Read the model definition and answer for the solid it produces. Units are mm, in the model's axes. A direction names the side the tool comes from. Give positions to 0.01 mm unless a question says otherwise; leave off trailing zeros. Write each loop counter-clockwise with the first axis right and the second up, starting at its lowest first coordinate (ties: lowest second). Pieces come first, ordered by that corner, then holes. Notation, with made-up numbers: (-28, 38.5) - (9, 38.5) arc R7 ccw to (9, 43.5) - close; hole circle Ø9 at (74.5, 78). An arc over 180 degrees is marked (long way). Answer as CSV lines item,"result".
Autodesk Inventor part; units mm, degrees
ref_plane "YZ Plane" through (0, 0, 0) normal (1, 0, 0) x (0, 1, 0)
ref_plane "XZ Plane" through (0, 0, 0) normal (0, 1, 0) x (-1, 0, 0)
ref_plane "XY Plane" through (0, 0, 0) normal (0, 0, 1) x (1, 0, 0)
sketch "Sketch1" plane through (0, 0, 0) normal (0, 0, 1) x (1, 0, 0)
  line L0 (-12.7529, 51.3281) -> (87.2471, 51.3281)
  line L1 (87.2471, 51.3281) -> (87.2471, -8.6719)
  line L2 (87.2471, -8.6719) -> (-12.7529, -8.6719)
  line L3 (-12.7529, -8.6719) -> (-12.7529, 51.3281)
  point P0 (0, 0)
  dimension "d0" = 100
  dimension "d1" = 60
extrude "Extrusion1" add sketch "Sketch1" along normal blind 40
shell "Shell1" thickness 2 removed faces 1 at (20.5805, 31.3281, 0)
sketch "Sketch2" plane through (85.2471, -6.6719, 38) normal (0, 0, -1) x (-1, 0, 0)
  line L0 (0, 0) -> (0, 56)
  line L1 (43.2, 19) -> (43.2, 37)
  line L2 (0, 37) -> (0, 19)
  line L3 (43.2, 19) -> (40.7, 19)
  line L4 (40.7, 19) -> (40.7, 22.5)
  line L5 (0, 16.6053) -> (0, 19)
  line L6 (0, 19) -> (2.5, 19)
  line L7 (2.5, 19) -> (2.5, 22.5)
  line L8 (2.5, 22.5) -> (40.7, 22.5)
  line L9 (0, 19) -> (2.5, 19)
  line L10 (40.7, 19) -> (43.2, 19)
  line L11 (43.2, 37) -> (40.7, 37)
  line L12 (40.7, 37) -> (40.7, 33.5)
  line L13 (40.7, 33.5) -> (2.5, 33.5)
  line L14 (2.5, 33.5) -> (2.5, 37)
  line L15 (43.2, 37) -> (40.7, 37)
  line L16 (2.5, 37) -> (0, 37)
  line L17 (96, 0) -> (0, 0)
  circle A0 centre (41.92, 20.3797) radius 0.9
  circle A1 centre (41.95, 35.62) radius 0.9
  circle A2 centre (1.28, 20.38) radius 0.9
  circle A3 centre (1.25, 35.62) radius 0.9
  line L18 (0, 56) -> (96, 56)
  point P0 (85.2471, 6.6719)
  point P1 (1.25, 19)
  point P2 (41.95, 19)
  point P3 (0, 37)
  point P4 (1.25, 37)
  point P5 (1.25, 19)
  dimension "d5" = 43.2
  dimension "d6" = 18
  dimension "d7" = 2.5
  dimension "d8" = 3.5
  dimension "d9" = 2.5
  dimension "d10" = 3.5
  dimension "d12" = 3.5
  dimension "d13" = 1.8
  dimension "d14" = 1.38
  dimension "d15" = 1.28
  dimension "d16" = 1.8
  dimension "d17" = 1.8
  dimension "d18" = 1.8
  dimension "d19" = 1.38
  dimension "d20" = 1.28
  dimension "d29" = 1.38
  dimension "d30" = 1.25
  dimension "d31" = 3.5
  dimension "d32" = 19
  dimension "d33" = 1.38
extrude "Extrusion2" add sketch "Sketch2" along normal blind 25
sketch "Sketch5" plane through (85.2471, -6.6719, 38) normal (0, 0, -1) x (-1, 0, 0)
  line L0 (0, 56) -> (96, 56)
  line L1 (77.9752, 56) -> (75.9752, 56)
  line L2 (75.9752, 56) -> (75.9752, 36)
  line L3 (75.9752, 36) -> (77.9752, 36)
  line L4 (77.9752, 36) -> (77.9752, 56)
  point P0 (85.2471, 6.6719)
  point P1 (75.9752, 56)
  dimension "d40" = 20
  dimension "d41" = 2
extrude "Extrusion5" add sketch "Sketch5" along normal blind 20
sketch "Sketch6" plane through (-12.7529, -8.6719, 0) normal (-1, 0, 0) x (0, 0, 1)
  circle A0 centre (27, 48) radius 3.5
  line L0 (18, 58) -> (18, 31.1645)
  line L1 (13, 23.2797) -> (38, 23.2797)
  line L2 (0, 58) -> (38, 58)
  point P0 (0, 8.6719)
  point P1 (18, 44.5822)
  dimension "d44" = 7
  dimension "d45" = 9
  dimension "d46" = 10
extrude "Extrusion6" cut sketch "Sketch6" against normal blind 4
sketch "Sketch7" plane through (-10.7529, -6.6719, 0) normal (1, 0, 0) x (0, 0, -1)
  circle A0 centre (-27, 46) radius 4.5
  line L0 (-40, -2) -> (-40, 58)
  circle A1 centre (-27, 46) radius 3.5
  line L1 (0, 56) -> (-38, 56)
  point P0 (0, 6.6719)
  dimension "d49" = 9
  dimension "d50" = 13
  dimension "d51" = 7
  dimension "d52" = 10
extrude "Extrusion7" add sketch "Sketch7" along normal blind 14
sketch "Sketch8" plane through (85.2471, -6.6719, 38) normal (0, 0, -1) x (-1, 0, 0)
  line L0 (96, 56) -> (96, 0)
  line L1 (96, 20.025) -> (76, 20.025)
  line L2 (76, 20.025) -> (76, 18.025)
  line L3 (76, 18.025) -> (96, 18.025)
  line L4 (96, 18.025) -> (96, 20.025)
  line L5 (96, 0) -> (0, 0)
  point P0 (85.2471, 6.6719)
  dimension "d55" = 20
  dimension "d56" = 2
  dimension "d57" = 18.025
extrude "Extrusion8" add sketch "Sketch8" along normal blind 20
sketch "Sketch9" plane through (-12.7529, -8.6719, 0) normal (0, -1, 0) x (1, 0, 0)
  circle A0 centre (12, 27) radius 3.5
  line L0 (0, 40) -> (100, 40)
  line L1 (2, 0) -> (2, 38)
  point P0 (12.7529, 0)
  dimension "d60" = 7
  dimension "d61" = 13
  dimension "d62" = 10
extrude "Extrusion9" cut sketch "Sketch9" against normal blind 4
sketch "Sketch10" plane through (-10.7529, -6.6719, 0) normal (0, 1, 0) x (1, 0, 0)
  circle A0 centre (10, -27) radius 3.5
  line L0 (98, -40) -> (-2, -40)
  line L1 (-2, 0) -> (-2, -40)
  circle A1 centre (10, -27) radius 4.5
  point P0 (10.7529, 0)
  dimension "d65" = 7
  dimension "d66" = 13
  dimension "d67" = 12
  dimension "d68" = 9
extrude "Extrusion10" add sketch "Sketch10" along normal blind 14
sketch "Sketch11" plane through (87.2471, -8.6719, 0) normal (1, 0, 0) x (0, 0, -1)
  line L0 (-5, 25.8) -> (-10, 25.8)
  line L1 (-10, 25.8) -> (-10, 34.2)
  line L2 (-10, 34.2) -> (-5, 34.2)
  line L3 (-5, 34.2) -> (-5, 25.8)
  line L4 (-40, 0) -> (-40, 60)
  line L5 (0, 0) -> (-40, 0)
  point P0 (0, 8.6719)
  dimension "d71" = 5
  dimension "d72" = 8.4
  dimension "d73" = 30
  dimension "d74" = 25.8
extrude "Extrusion11" cut sketch "Sketch11" against normal blind 2
sketch "Sketch12" plane through (85.2471, -6.6719, 38) normal (0, 0, -1) x (-1, 0, 0)
  line L0 (96, 0) -> (0, 0)
  line L1 (96, 0) -> (93, 0)
  line L2 (93, 0) -> (93, 1)
  line L3 (95, 3) -> (96, 3)
  line L4 (96, 3) -> (96, 0)
  line L5 (96, 56.0056) -> (93, 56.0056)
  line L6 (93, 56.0056) -> (93, 55.0056)
  line L7 (95, 53.0056) -> (96, 53.0056)
  line L8 (96, 53.0056) -> (96, 56.0056)
  line L9 (0, 56.0056) -> (3, 56.0056)
  line L10 (3, 56.0056) -> (3, 55.0056)
  line L11 (1, 53.0056) -> (0, 53.0056)
  line L12 (0, 53.0056) -> (0, 56.0056)
  line L13 (0, 0) -> (3, 0)
  line L14 (3, 0) -> (3, 1)
  line L15 (1, 3) -> (0, 3)
  line L16 (0, 3) -> (0, 0)
  circle A0 centre (95, 55.0056) radius 1
  arc A1 (93, 55.0056) -> (95, 53.0056) centre (95, 55.0056) ccw
  arc A2 (95, 3) -> (93, 1) centre (95, 1) ccw
  arc A3 (1, 53.0056) -> (3, 55.0056) centre (1, 55.0056) ccw
  arc A4 (3, 1) -> (1, 3) centre (1, 1) ccw
  circle A5 centre (95, 1) radius 1
  circle A6 centre (1, 1) radius 1
  circle A7 centre (1, 55.0056) radius 1
  point P0 (85.2471, 6.6719)
  point P1 (93, 3)
  point P2 (93, 53.0056)
  point P3 (3, 53.0056)
  point P4 (3, 3)
  point P5 (0, 1)
  point P6 (1, 0)
  point P7 (3, 0)
  point P8 (1, 56.0056)
  point P9 (0, 55.0056)
  point P10 (95, 56.0056)
  point P11 (96, 55.0056)
  point P12 (96, 1)
  point P13 (95, 0)
  dimension "d77" = 3
  dimension "d78" = 3
  dimension "d79" = 3
  dimension "d80" = 3
  dimension "d81" = 3
  dimension "d82" = 3
  dimension "d83" = 3
  dimension "d84" = 2
  dimension "d85" = 0
  dimension "d86" = 1
  dimension "d87" = 2
  dimension "d88" = 2
  dimension "d89" = 2
  dimension "d90" = 2
extrude "Extrusion12" add sketch "Sketch12" along normal blind 38 contours L0 A6 L16 L15 A4 L14 | L2 A2 L3 L4 A5 L0 | A5 L4 L0 | L0 L16 A6 | L8 A0 L5 | A0 L8 L7 A1 L6 L5 | L9 A7 L12 | L9 L10 A3 L11 L12 A7
sketch "Sketch13" plane through (-12.7529, 51.3281, 0) normal (0, 1, 0) x (1, 0, 0)
  line L0 (35.7867, -12.2294) -> (42.7867, -12.2294)
  line L1 (42.7867, -12.2294) -> (42.7867, -5.2294)
  line L2 (42.7867, -5.2294) -> (35.7867, -5.2294)
  line L3 (35.7867, -5.2294) -> (35.7867, -12.2294)
  point P0 (12.7529, 0)
  dimension "d93" = 7
  dimension "d94" = 7
extrude "Extrusion13" cut sketch "Sketch13" against normal blind 10
(1) The mould has two halves that part along X. Classify faces 1 (the flat face through (38, -8.672, 20)), 2 (the flat face through (64, 15.828, 26)): +X half, -X half, draft (parallel to the pull), parting line (faces both ways), or undercut.
Worked out:
face 1,"draft"
face 2,"undercut"
(2) A cutting plane is placed at D-D (z = 27). Count the separate pieces of the cut face and the enclosed holes in it, and give its area (3 significant figures).
Worked out:
separate pieces,"2"
enclosed holes,"8"
area,"1,250 mm^2"
(3) Each of these flat-tipped pins is pushed along its axis until it touches: P1, Ø1.6, axis at x = 8.5, y = 44, coming from the -Z side; P2, Ø1.5, axis at x = 1.5, y = 5, coming from the -Z side; P3, Ø2, axis at x = 43, y = 14, coming from the -Z side. Where does it stop, or does it pass through?
Worked out:
P1,"stops at z = 18"
P2,"stops at z = 22.76"
P3,"stops at z = 13"
(4) A cutting plane is placed at C-C (y = 23). Write down the section's boundary in (x, z).
Worked out:
outline,"(-12.75, 0) - (-10.75, 0) - (-10.75, 38) - (42.05, 38) - (42.05, 13) - (85.25, 13) - (85.25, 10) - (87.25, 10) - (87.25, 40) - (-12.75, 40) - close; (85.25, 0) - (87.25, 0) - (87.25, 5) - (85.25, 5) - close"
(5) A cutting plane is placed at A-A (y = 1.5). Write down the section's boundary in (x, z).
Worked out:
outline,"(-12.75, 0) - (-10.75, 0) - (-10.75, 38) - (85.25, 38) - (85.25, 0) - (87.25, 0) - (87.25, 40) - (-12.75, 40) - close; circle Ø9 at (-0.75, 27); hole circle Ø7 at (-0.75, 27)"
(6) For faces 3 (the cylindrical face through (1.67, 0.23, 30.79)), 4 (the flat face through (86, 25.528, 8)), 5 (the flat face through (30.034, 50, 9)), 6 (the flat face through (9.272, 39, 28)), determine the directions among +Z, -Z, +X, -X, +Y, -Y from which every point of the face is accessible in a straight line to the end or side of a thin tool.
Worked out:
face 3,"none"
face 4,"+X"
face 5,"+Y"
face 6,"-Z"
(7) A cutting plane is placed at B-B (x = 28). Write down the section's boundary in (y, z), and give its area (3 significant figures).
Worked out:
outline,"(-8.67, 0) - (-6.67, 0) - (-6.67, 38) - (49.33, 38) - (49.33, 12.23) - (51.33, 12.23) - (51.33, 40) - (-8.67, 40) - close; (49.33, 0) - (51.33, 0) - (51.33, 5.23) - (49.33, 5.23) - close"
area,"258 mm^2"
(8) Find the intervals of material crossed by L1, parallel to Y at x = 81, z = 18; L2, parallel to Y at x = -0.75, z = 27; L3, parallel to X at y = 42, z = 23, in increasing order.
Worked out:
L1,"y = -8.67 to -6.67, 15.83 to 26.83, 49.33 to 51.33"
L2,"y = 11.35 to 13.35, 34.83 to 35.83, 42.83 to 43.83, 49.33 to 51.33"
L3,"x = -12.75 to -10.75, 7.27 to 9.27, 85.25 to 87.25"
